Design review of the part built by this model. Coordinates are the model's own, in mm. A direction names the side the tool comes from. Coordinates: 2 decimals unless noted, no trailing zeros. Write each loop counter-clockwise with the first axis right and the second up, starting at its lowest first coordinate (ties: lowest second). Pieces come first, ordered by that corner, then holes.
Q1. The part is to be moulded in two halves that separate along X. For faces 1 (the face through (-1.13, -3.13, 14.35)), 2 (the face through (16.024, -5.046, 7.37)), 3 (the face through (-8, -12, 0)), say which applies: +X half, -X half, draft (parallel to the pull), parting line (faces both ways), or undercut.
Q2. Clearance check with flat-ended pins moving along their axes: pin 1 Ø3 at (y, z) = (-9.5, 10.5) entering from -X; pin 2 Ø6 at (x, y) = (-5, 0) entering from +Z; pin 3 Ø3 at (y, z) = (-9, 2.5) entering from +X. State where each tip first meets the part, or that it passes through.
Q3. Machinability: for faces 4 (the face through (2.58, 4.05, 9.96)), 5 (the face through (-8, -12, 14.95)), 6 (the face through (0, 0, 2.5)), which of the approach directions +Z, -Z, +X, -X, +Y, -Y give a long, thin tool a straight path to every point of the face, cutting with its end or side? Answer none if there is none.
Q4. Add section D-D, the plane z = 2. Give the boundary of the cut face in (x, y), plus the area to 3 significant figures.
Q5. Add section A-A, the plane x = 0. Give the boundary of the cut face in (y, z) (3 decimals).
Q6. To check wall thickness, follow probe 1 along Y at (x, z) = (0, 9.75) (3 decimals); probe 2 along Y at (x, z) = (0, 5.5) (3 decimals); probe 3 along Y at (x, z) = (0, 2). State the ranges of each line that lie inside material, in increasing order.
Q7. Add section C-C, the plane z = 8.75. Give the boundary of the cut face in (x, y) (3 decimals).
Autodesk Inventor part; units mm, degrees
ref_plane "YZ Plane" through (0, 0, 0) normal (1, 0, 0) x (0, 1, 0)
ref_plane "XZ Plane" through (0, 0, 0) normal (0, 1, 0) x (-1, 0, 0)
ref_plane "XY Plane" through (0, 0, 0) normal (0, 0, 1) x (1, 0, 0)
sketch "Esboço1" plane through (0, 0, 0) normal (0, 0, 1) x (1, 0, 0)
  circle A0 centre (0, 0) radius 16.8
  dimension "d0" = 33.6
extrude "Extrusão1" add sketch "Esboço1" along normal blind 14.95
sketch "Esboço6" plane through (0, 0, 0) normal (0, 0, -1) x (-1, 0, 0)
  circle A0 centre (0, 0) radius 14.25
  dimension "d15" = 28.5
extrude "Extrusão6" cut sketch "Esboço6" against normal blind 2.5
sketch "Esboço7" plane through (0, 0, 14.95) normal (0, 0, 1) x (1, 0, 0)
  circle A0 centre (0, 0) radius 14.25
  circle A1 centre (0, 0) radius 4.8
  dimension "d18" = 28.5
  dimension "d19" = 9.6
extrude "Extrusão7" cut sketch "Esboço7" against normal blind 9.5
sketch "Esboço8" plane through (0, 0, 14.95) normal (0, 0, 1) x (1, 0, 0)
  circle A0 centre (0, 0) radius 4.8
extrude "Extrusão8" cut sketch "Esboço8" against normal blind 0.6
sketch "Esboço9" plane through (0, 0, 14.35) normal (0, 0, 1) x (1, 0, 0)
  circle A0 centre (0, 0) radius 4.8
  circle A1 centre (0, 0) radius 3.175
  dimension "d24" = 6.35
extrude "Extrusão9" cut sketch "Esboço9" against normal blind 7.9 contours A1
sketch "Esboço10" plane through (0, 0, 6.45) normal (0, 0, 1) x (1, 0, 0)
  circle A0 centre (0, 0) radius 1.175
  dimension "d27" = 2.35
extrude "Extrusão10" cut sketch "Esboço10" against normal blind 1.75
chamfer "Chanfro1" distance 0.25 angle 45 1 edges at (-1.175, 0, 6.45)
properties part number "roda"
Here are the results:
1. face 1: undercut
1. face 2: parting line
1. face 3: draft
2. pin 1: stops at x = -14.77
2. pin 2: stops at z = 14.35
2. pin 3: stops at x = 15.03
3. face 4: +Z
3. face 5: +Z, +X, -X, +Y, -Y
3. face 6: -Z
4. outline: circle Ø33.6 at (0, 0); hole circle Ø28.5 at (0, 0)
4. area: 249 mm2
5. outline: (-16.8, 0) - (-14.25, 0) - (-14.25, 2.5) - (14.25, 2.5) - (14.25, 0) - (16.8, 0) - (16.8, 14.95) - (14.25, 14.95) - (14.25, 5.45) - (4.8, 5.45) - (4.8, 14.35) - (3.175, 14.35) - (3.175, 6.45) - (1.425, 6.45) - (1.175, 6.2) - (1.175, 4.7) - (-1.175, 4.7) - (-1.175, 6.2) - (-1.425, 6.45) - (-3.175, 6.45) - (-3.175, 14.35) - (-4.8, 14.35) - (-4.8, 5.45) - (-14.25, 5.45) - (-14.25, 14.95) - (-16.8, 14.95) - close
6. probe 1: y = -16.8 to -14.25, -4.8 to -3.175, 3.175 to 4.8, 14.25 to 16.8
6. probe 2: y = -16.8 to -14.25, -4.8 to -1.175, 1.175 to 4.8, 14.25 to 16.8
6. probe 3: y = -16.8 to -14.25, 14.25 to 16.8
7. outline: circle Ø33.6 at (0, 0); circle Ø9.6 at (0, 0); hole circle Ø28.5 at (0, 0); hole circle Ø6.35 at (0, 0)
